from build123d import *

# Parameters (mm, degrees)
CROQUIS1_R              = 1
SALIENTE_EXTRUIR1_DEPTH = 1.7


with BuildPart() as part:
    # Croquis1 → Saliente-Extruir1 (new body)
    with BuildSketch(Plane.XY):
        with BuildLine():
            Line((-2.5, 10.1), (-10.1, 10.1))
            Line((-10.1, 10.1), (-10.1, 2))
            ThreePointArc((-10.1, 2), (-12.1, 0), (-10.1, -2))
            Line((-10.1, -2), (-10.1, -10.1))
            Line((-10.1, -10.1), (-2.5, -10.1))
            ThreePointArc((-2.5, -10.1), (0, -7.6), (2.5, -10.1))
            Line((2.5, -10.1), (10.1, -10.1))
            Line((10.1, -10.1), (10.1, -2))
            ThreePointArc((10.1, -2), (12.1, 0), (10.1, 2))
            Line((10.1, 2), (10.1, 10.1))
            Line((10.1, 10.1), (2.5, 10.1))
            ThreePointArc((2.5, 10.1), (0, 7.6), (-2.5, 10.1))
        make_face()
        with Locations((-10.1, 0)):
            Circle(CROQUIS1_R, mode=Mode.SUBTRACT)
        with Locations((10.1, 0)):
            Circle(CROQUIS1_R, mode=Mode.SUBTRACT)
    extrude(amount=SALIENTE_EXTRUIR1_DEPTH)


solid = part.part
Work out the finished part from the listing and answer in its coordinate system (mm). A direction names the side the tool comes from. Round coordinates to 2 decimals unless told otherwise and drop trailing zeros. Order: outer loops, then holes, each group sorted by start corner. A loop starts at its lowest first (then second) coordinate and runs counter-clockwise, first axis right, second up. Notation, with made-up numbers: M -19.5,26 L 26.5,26 A22 ccw 26.5,46 Z; hole C 16,23 d9. An arc over 180 degrees is marked long. One line per item, written item: value.
Q1. Flat-ended cylindrical pins translate along their axes: pin 1 (1.2 mm diameter, centred on x = -10.1, y = 0, fed in from -Z); pin 2 (1 mm diameter, centred on x = -1, z = 0.5, fed in from +Y). Find the tip coordinate at first contact, or state that the pin passes through.
Derived:
pin 1: through
pin 2: y = 8.1
Q2. Determine the mould class of faces 4 (the face through (-10.1, -6, 1)), 5 (the face through (-11.1, 0, 0.8)), 6 (the face through (-12.1, 0, 0.8)) for opening direction Y: released by +Y, released by -Y, zero draft, split by the parting line, or undercut.
Derived:
face 4: zero draft
face 5: undercut
face 6: split by the parting line
Q3. Straight lines are drawn through the part: line 1 (X direction, y = 0.75, z = 1.5); line 2 (X direction, y = 7.5, z = 1.35); line 3 (X direction, y = -8.25, z = 0.4). For each, find the intervals that lie inside material, in ascending order.
Derived:
line 1: -11.95 to -10.76, -9.44 to 9.44, 10.76 to 11.95
line 2: -10.1 to 10.1
line 3: -10.1 to -1.68, 1.68 to 10.1
Q4. Find section C-C on x = 9.75. Write down the section's boundary in (y, z), then the cut area to 3 significant figures.
Derived:
outline: M -10.1,0 L -0.94,0 L -0.94,1.7 L -10.1,1.7 Z; M 0.94,0 L 10.1,0 L 10.1,1.7 L 0.94,1.7 Z
area: 31.2 mm²
Q5. For faces 1 (the face through (10.1, 6, 1)), 2 (the face through (-10.1, 6, 1)), 3 (the face through (10.1, -6, 1)), determine the directions among +Z, -Z, +X, -X, +Y, -Y from which every point of the face is accessible in a straight line to the end or side of a thin tool.
Derived:
face 1: +Z, -Z, +X, +Y
face 2: +Z, -Z, -X, +Y
face 3: +Z, -Z, +X, -Y
Q6. Find section A-A on y = 0. Write down the section's boundary in (x, z).
Derived:
outline: M -12.1,0 L -11.1,0 L -11.1,1.7 L -12.1,1.7 Z; M -9.1,0 L 9.1,0 L 9.1,1.7 L -9.1,1.7 Z; M 11.1,0 L 12.1,0 L 12.1,1.7 L 11.1,1.7 Z
Q7. Find section D-D on y = -3. Write down the section's boundary in (x, z), then the cut area to 3 significant figures.
Derived:
outline: M -10.1,0 L 10.1,0 L 10.1,1.7 L -10.1,1.7 Z
area: 34.3 mm²
Q8. Find section B-B on z = 0.4. Write down the section's boundary in (x, y), then the cut area to 3 significant figures.
Derived:
outline: M -10.1,-10.1 L -2.5,-10.1 A2.5 cw 2.5,-10.1 L 10.1,-10.1 L 10.1,-2 A2 ccw 10.1,2 L 10.1,10.1 L 2.5,10.1 A2.5 cw -2.5,10.1 L -10.1,10.1 L -10.1,2 A2 ccw -10.1,-2 Z; hole C -10.1,0 d2; hole C 10.1,0 d2
area: 395 mm²
